from build123d import *

# Parameters (mm, degrees)
BOSS_EXTRUDE1_DEPTH = 152.5
SKETCH9_R           = 35
CUT_EXTRUDE1_DEPTH  = 152.5


with BuildPart() as part:
    # Sketch1 → Boss-Extrude1 (new body)
    # profile 1 of 2: a face of its own
    with BuildSketch(Plane(origin=(0, 0, 0), x_dir=(1, 0, 0), z_dir=(0, 1, 0))):
        with BuildLine():
            Line((300, 0), (140.492545905, 0))
            Line((140.492545905, 0), (0, -140.492545905))
            Line((0, -140.492545905), (0, -237.5))
            Line((0, -237.5), (161.5, -237.5))
            ThreePointArc((161.5, -237.5), (259.434289194, -196.934289194), (300, -99))
            Line((300, -99), (300, 0))
        make_face()
        with BuildLine():
            Line((245.352869941, -70.987750493), (121.920310217, -194.420310217))
            ThreePointArc((121.920310217, -194.420310217), (78.079689783, -194.420310217), (78.079689783, -150.579689783))
            Line((78.079689783, -150.579689783), (201.512249507, -27.147130059))
            ThreePointArc((201.512249507, -27.147130059), (245.352869941, -27.147130059), (245.352869941, -70.987750493))
        make_face(mode=Mode.SUBTRACT)
    # profile 2 of 2: a face of its own
    with BuildSketch(Plane(origin=(0, 0, 0), x_dir=(1, 0, 0), z_dir=(0, 1, 0))):
        with BuildLine():
            Line((0, 237.5), (0, 140.492545905))
            Line((0, 140.492545905), (140.492545905, 0))
            Line((140.492545905, 0), (300, 0))
            Line((300, 0), (300, 99))
            ThreePointArc((300, 99), (259.434289194, 196.934289194), (161.5, 237.5))
            Line((161.5, 237.5), (0, 237.5))
        make_face()
        with BuildLine():
            ThreePointArc((78.079689783, 150.579689783), (78.079689783, 194.420310217), (121.920310217, 194.420310217))
            Line((121.920310217, 194.420310217), (245.352869941, 70.987750493))
            ThreePointArc((245.352869941, 70.987750493), (245.352869941, 27.147130059), (201.512249507, 27.147130059))
            Line((201.512249507, 27.147130059), (78.079689783, 150.579689783))
        make_face(mode=Mode.SUBTRACT)
    extrude(amount=BOSS_EXTRUDE1_DEPTH)

    # Sweep2: sweep along a path in Sketch2
    with BuildLine(Plane.XY) as sweep2_path:
        Line((300, 152.5), (345.356342374, 152.5))
        ThreePointArc((345.356342374, 152.5), (416.313076896, 140.45354598), (479.318397094, 105.664110009))
        Line((479.318397094, 105.664110009), (641.03794528, -23.164110009))
        ThreePointArc((641.03794528, -23.164110009), (704.043265478, -57.95354598), (775, -70))
        Line((775, -70), (1000, -70))
    # Sketch3 → Sweep2 (sweep)
    with BuildSketch(Plane(origin=(300, 0, 0), x_dir=(0, 0, -1), z_dir=(1, 0, 0))):
        Polygon((-37.5, 152.5), (37.5, 152.5), (37.5, 132.5), (10, 132.5), (10, 72.5), (37.5, 72.5), (37.5, 52.5), (-37.5, 52.5), (-37.5, 72.5), (-10, 72.5), (-10, 132.5), (-37.5, 132.5), align=None)
    sweep(path=sweep2_path.line)

    # Sketch7 → Revolve2 (revolve)
    with BuildSketch(Plane(origin=(0, 0, 0), x_dir=(-1, 0, 0), z_dir=(0, 0, -1))):
        Polygon((-920, -70), (-920, -90), (-990, -90), (-990, -150), (-920.012979842, -150), (-920.012979842, -168.558956517), (-1000, -170), (-1000, -70), align=None)
    revolve(axis=Axis((1000, -43.921847772, 0), (0, -1, 0)))

    # Sketch9 → Cut-Extrude1 (cut)
    with BuildSketch(Plane(origin=(0, -70, 0), x_dir=(1, 0, 0), z_dir=(0, 1, 0))):
        with Locations(Location((1000, 0, 0), (0, 0, 180))):
            Circle(SKETCH9_R)
    extrude(amount=-CUT_EXTRUDE1_DEPTH, mode=Mode.SUBTRACT)


solid = part.part
For this review, take the finished solid that the model builds, in its own axes (mm). A direction names the side the tool comes from. Round coordinates to 2 decimals unless told otherwise and drop trailing zeros. Order: outer loops, then holes, each group sorted by start corner. A loop starts at its lowest first (then second) coordinate and runs counter-clockwise, first axis right, second up. Notation, with made-up numbers: (19, -33) -> (52, -33) arc R17 ccw to (52, -15) -> close; hole circle Ø4 at (11, -39.75). An arc over 180 degrees is marked (long way). Put each result on its own line as item: value.
Q1. Machinability: for faces 1 (the flat face through (69.26, 75.18, -71.23)), 2 (the cylindrical face through (389.31, 65.144, -23.557)), 3 (the flat face through (925, -150, -19)), 4 (the flat face through (323, 132.5, 24)), 5 (the flat face through (323, 52.5, 1)), which of the approach directions +Z, -Z, +X, -X, +Y, -Y give a long, thin tool a straight path to every point of the face, cutting with its end or side? Answer none if there is none.
Check result:
face 1: -X, +Y, -Y
face 2: -Z
face 3: +X
face 4: +Z
face 5: +Z, -Z, -Y
Q2. Insertion check: pin 1 Ø4 at (x, z) = (132.5, -55.5) entering from -Y; pin 2 Ø8 at (x, z) = (330.5, -20) entering from -Y; pin 3 Ø4 at (x, y) = (886.5, -90.5) entering from +Z. Each pin has a flat end and moves straight along its axis. Give the tip position at first contact, or say it passes through.
Check result:
pin 1: y = 0
pin 2: y = 52.5
pin 3: z = 37.5
Q3. For probe 1 along Y at (x, z) = (283, 12.5); probe 2 along Z at (x, y) = (760, -98); probe 3 along X at (y, z) = (37.5, -119), list the stretches that pass through material, from the lowest coordinate up. Write a range as [from, to].
Check result:
probe 1: [0, 152.5]
probe 2: [-10, 10]
probe 3: [21.49, 109.66], [197.34, 298.55]
Q4. Add section C-C on y = -11.5. Write out the cut boundary in (x, z).
Check result:
outline: (465.9, -37.5) -> (498, -37.5) -> (498, -10) -> (594.3, -10) -> (594.3, -37.5) -> (626.4, -37.5) -> (626.4, 37.5) -> (594.3, 37.5) -> (594.3, 10) -> (498, 10) -> (498, 37.5) -> (465.9, 37.5) -> close
Q5. Mouldability with a two-part tool opening along X and no side actions: class faces 6 (the flat face through (80, 75, 237.5)), 7 (the cylindrical face through (415.357, 140.785, 0.525)), 8 (the flat face through (635, -51, -10)) as pulls with the +X half, pulls with the -X half, needs draft (parallel to the pull), parting line crosses it, or undercut.
Check result:
face 6: needs draft
face 7: pulls with the +X half
face 8: undercut
Q6. Add section A-A on z = -121.5. Write out the cut boundary in (x, y).
Check result:
outline: (18.99, 0) -> (107.16, 0) -> (107.16, 152.5) -> (18.99, 152.5) -> close; (194.84, 0) -> (298.16, 0) -> (298.16, 152.5) -> (194.84, 152.5) -> close
Q7. Add section B-B on x = 100. Write out the cut boundary in (y, z), plus the area to 3 significant figures.
Check result:
outline: (0, -237.5) -> (152.5, -237.5) -> (152.5, -203.5) -> (0, -203.5) -> close; (0, -128.66) -> (152.5, -128.66) -> (152.5, -40.49) -> (0, -40.49) -> close; (0, 40.49) -> (152.5, 40.49) -> (152.5, 128.66) -> (0, 128.66) -> close; (0, 203.5) -> (152.5, 203.5) -> (152.5, 237.5) -> (0, 237.5) -> close
area: 37,300 mm2
Q8. Add section D-D on z = -172.5. Write out the cut boundary in (x, y).
Check result:
outline: (0, 0) -> (69, 0) -> (69, 152.5) -> (0, 152.5) -> close; (143.84, 0) -> (278.89, 0) -> (278.89, 152.5) -> (143.84, 152.5) -> close
